Here's how the part is built. I have some questions about the finished solid (model axes, mm). Face numbers are marked on the shaded views. A direction names the side the tool comes from. Give positions to 0.01 mm unless a question says otherwise; leave off trailing zeros. Loops run counter-clockwise (first coordinate to the right, second up) from the corner with the lowest first, then second, coordinate; pieces in that order, holes last. Notation, with made-up numbers: (-10, -25) - (-6, -25) arc R21 ccw to (-6, -19) - close; hole circle Ø5 at (27.5, -7.5). An arc over 180 degrees is marked (long way). Put each result on its own line as item: value. Start each with the question number.
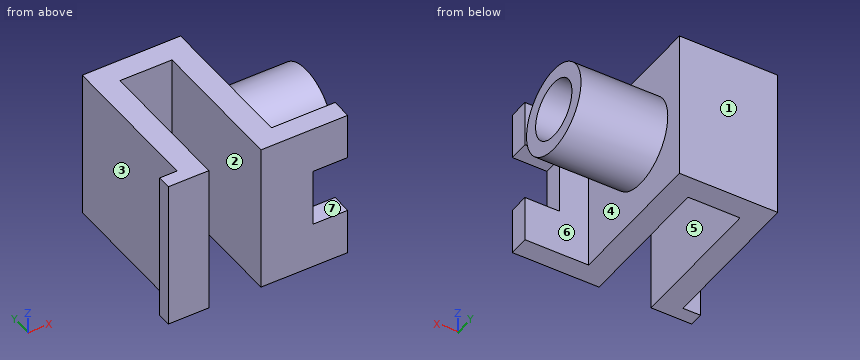
from build123d import *

# Parameters (mm, degrees)
SALIENTE_EXTRUIR2_DEPTH = 26
CORTAR_EXTRUIR1_DEPTH   = 84.785440263
CROQUIS4_R              = 15
CROQUIS4_R_2            = 10
SALIENTE_EXTRUIR3_DEPTH = 30


with BuildPart() as part:
    # Croquis1 → Saliente-Extruir2 (new, symmetric)
    with BuildSketch(Plane.XY):
        Polygon((0, 0), (14, 0), (14, 49), (32, 49), (32, 0), (62, 0), (62, 7), (40, 7), (40, 57), (6, 57), (6, 4.804511278), (0, 4.804511278), align=None)
    extrude(amount=SALIENTE_EXTRUIR2_DEPTH, both=True)

    # Croquis3 → Cortar-Extruir1 (cut, through all)
    with BuildSketch(Plane(origin=(0, 7, 0), x_dir=(1, 0, 0), z_dir=(0, 1, 0))):
        Polygon((62, 0), (62, 10), (50, 10), (50, -10), (62, -10), align=None)
    extrude(amount=-CORTAR_EXTRUIR1_DEPTH, mode=Mode.SUBTRACT)

    # Croquis4 → Saliente-Extruir3 (add)
    with BuildSketch(Plane(origin=(40, 0, 0), x_dir=(0, 0, -1), z_dir=(1, 0, 0))):
        with Locations(Location((0, 35.609925513, 0), (0, 0, 180))):
            Circle(CROQUIS4_R)
        with Locations((0, 35.609925513)):
            Circle(CROQUIS4_R_2, mode=Mode.SUBTRACT)
    extrude(amount=SALIENTE_EXTRUIR3_DEPTH)


solid = part.part
1) Suppose I cut it at D-D on x = 28. Please give me the cut outline in (y, z), plus the area to 3 significant figures.
2) Suppose I cut it at A-A on y = 15. Please give me the cut outline in (x, z), plus the area to 3 significant figures.
3) Thinking about a two-plate mould opening in X: for the marked faces 1, 2 and 3, which applies, pulls with the +X half, pulls with the -X half, needs draft (parallel to the pull), parting line crosses it, or undercut?
4) Suppose I cut it at C-C on z = 0. Please give me the cut outline in (x, y).
5) I'm going to push flat-ended pins straight in: P1, Ø10, axis at y = 39, z = -3.5, coming from the +X side; P2, Ø10, axis at y = 26.5, z = -3.5, coming from the -X side; P3, Ø5.5, axis at y = 2, z = -2, coming from the +X side. Where does each tip first touch, or does it pass through?
6) Suppose I cut it at B-B on x = 61. Please give me the cut outline in (y, z).
7) I need wall thicknesses on line 1 (X direction, y = 37, z = 12); line 2 (Y direction, x = 52.5, z = 0.5); line 3 (X direction, y = 19, z = 10.5). Which ranges of each line are inside material? Lowest first, please.
8) Which directions (+Z, -Z, +X, -X, +Y, -Y) give clear straight access to the entire face, cutting with the end or side of a thin tool? Please do the marked faces 4, 5, 6 and 7.
Ans:
1. outline: (49, -26) - (57, -26) - (57, 26) - (49, 26) - close
1. area: 416 mm²
2. outline: (6, -26) - (14, -26) - (14, 26) - (6, 26) - close; (32, -26) - (40, -26) - (40, 26) - (32, 26) - close
2. area: 832 mm²
3. face 1: needs draft
3. face 2: undercut
3. face 3: pulls with the -X half
4. outline: (0, 0) - (14, 0) - (14, 49) - (32, 49) - (32, 0) - (50, 0) - (50, 7) - (40, 7) - (40, 20.61) - (70, 20.61) - (70, 25.61) - (40, 25.61) - (40, 45.61) - (70, 45.61) - (70, 50.61) - (40, 50.61) - (40, 57) - (6, 57) - (6, 4.8) - (0, 4.8) - close
5. P1: stops at x = 40
5. P2: stops at x = 6
5. P3: stops at x = 50
6. outline: (0, -26) - (7, -26) - (7, -10) - (0, -10) - close; (0, 10) - (7, 10) - (7, 26) - (0, 26) - close; circle Ø30 at (35.61, 0); hole circle Ø20 at (35.61, 0)
7. line 1: x = 6 to 14, 32 to 70
7. line 2: y = 20.62 to 25.62, 45.6 to 50.6
7. line 3: x = 6 to 14, 32 to 40
8. face 4: +X
8. face 5: +Z, -Z, -Y
8. face 6: +Z, -Z, +X
8. face 7: +X, -Y
